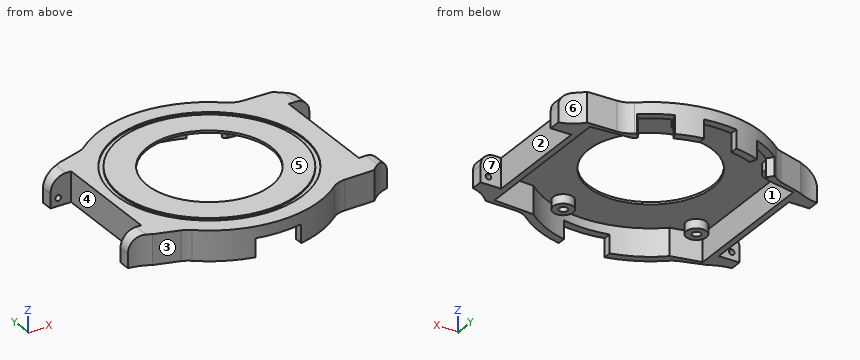
```python
from build123d import *

# Parameters (mm, degrees)
PAD_DEPTH       = 6.5
POCKET_DEPTH    = 6
SKETCH002_R     = 13.5
POCKET001_DEPTH = 1
SKETCH003_W     = 5.4
SKETCH003_H     = 6.5
PAD001_DEPTH    = 4.5
POCKET002_DEPTH = 10
SKETCH008_R     = 0.6
POCKET003_DEPTH = 2
SKETCH009_R     = 0.6
POCKET004_DEPTH = 2
FILLET_R        = 2.9
FILLET001_R     = 2.9
FILLET002_R     = 5
FILLET003_R     = 5
FILLET004_R     = 5
FILLET005_R     = 5
SKETCH010_W     = 3.95
SKETCH010_H     = 6.5
PAD002_DEPTH    = 4.5
POCKET005_DEPTH = 10
SKETCH012_R     = 0.6
POCKET006_DEPTH = 2
SKETCH013_R     = 0.6
POCKET007_DEPTH = 2
FILLET006_R     = 3.4
FILLET007_R     = 3.4
SKETCH014_R     = 20.45
SKETCH014_R_2   = 19.5
POCKET008_DEPTH = 0.3
SKETCH015_R     = 2.2
SKETCH015_R_2   = 0.925
PAD003_DEPTH    = 2
POCKET009_DEPTH = 4
POCKET010_DEPTH = 4


with BuildPart() as part:
    # Sketch → Pad (new body)
    with BuildSketch(Plane.XY):
        with BuildLine():
            Line((-22.5019915649, 16), (-22.5019915649, -16))
            Line((-22.5019915649, -16), (-16.2858834578, -17.9000000001))
            ThreePointArc((-16.2858834577, -17.9000000001), (0.2206895737, -24.1989937004), (16.6096357576, -17.5999999999))
            Line((16.6096357576, -17.5999999999), (24.9082802252, -17.45))
            Line((24.9082802252, 17.45), (24.9082802252, -17.45))
            Line((16.6096357576, 17.6), (24.9082802252, 17.45))
            ThreePointArc((16.6096357576, 17.6), (0.2206895736, 24.1989937004), (-16.2858834578, 17.9))
            Line((-22.5019915649, 16), (-16.2858834578, 17.9))
        make_face()
    extrude(amount=PAD_DEPTH)

    # Sketch001 → Pocket (cut)
    with BuildSketch(Plane.XY):
        with BuildLine():
            Line((-14.8539557021, 16.9), (-21.2122180433, 15.55))
            Line((-21.2122180433, 15.55), (-21.2122180433, -15.55))
            Line((-21.2122180433, -15.55), (-14.8539557021, -16.9))
            ThreePointArc((-14.8539557021, -16.9), (-0.0760301383, -22.4998715423), (14.739402973, -17))
            Line((14.739402973, -17), (23.6191552218, -16.4))
            Line((23.6191552218, 16.4), (23.6191552218, -16.4))
            Line((14.739402973, 17), (23.6191552218, 16.4))
            ThreePointArc((14.739402973, 17), (-0.0760301383, 22.4998715423), (-14.8539557021, 16.9))
        make_face()
    extrude(amount=POCKET_DEPTH, mode=Mode.SUBTRACT)

    # Sketch002 (on Face19 of Pocket) → Pocket001 (cut)
    with BuildSketch(Plane(origin=(0, 0, 6), x_dir=(1, 0, 0), z_dir=(0, 0, -1))):
        Circle(SKETCH002_R)
    extrude(amount=-POCKET001_DEPTH, mode=Mode.SUBTRACT)

    # Sketch003 (on Face6 of Pocket001) → Pad001 (join)
    with BuildSketch(Plane.YZ.offset(24.9082802252)):
        with Locations((-14.75, 3.25)):
            Rectangle(SKETCH003_W, SKETCH003_H)
        with Locations((14.75, 3.25)):
            Rectangle(SKETCH003_W, SKETCH003_H)
    extrude(amount=PAD001_DEPTH)

    # Sketch006 → Pocket002 (cut)
    with BuildSketch(Plane.XY.offset(6.5)):
        with BuildLine():
            ThreePointArc((24.9082802253, 17.45), (26.9423471239, 15.7065020586), (29.4082802252, 14.6594169812))
            Line((29.4082802252, 17.45), (29.4082802252, 14.6594169812))
            Line((29.4082802252, 17.45), (24.9082802252, 17.45))
        make_face()
        with BuildLine():
            ThreePointArc((29.4082802253, -14.6594169812), (26.9423471239, -15.7065020586), (24.9082802253, -17.45))
            Line((29.4082802252, -17.45), (24.9082802252, -17.45))
            Line((29.4082802253, -14.6594169811), (29.4082802252, -17.45))
        make_face()
    extrude(amount=-POCKET002_DEPTH, mode=Mode.SUBTRACT)

    # Sketch008 (on Face27 of Pocket002) → Pocket003 (cut)
    with BuildSketch(Plane(origin=(0, -12.05, 0), x_dir=(-1, 0, 0), z_dir=(0, 1, 0))):
        with Locations((-27.7082802252, 1.7)):
            Circle(SKETCH008_R)
    extrude(amount=-POCKET003_DEPTH, mode=Mode.SUBTRACT)

    # Sketch009 (on Face26 of Pocket003) → Pocket004 (cut)
    with BuildSketch(Plane.XZ.offset(-12.05)):
        with Locations((27.7082802252, 1.7)):
            Circle(SKETCH009_R)
    extrude(amount=-POCKET004_DEPTH, mode=Mode.SUBTRACT)

    # Fillet
    fillet_edges = [part.edges().sort_by_distance(p)[0] for p in [
        (29.40828, -13.354708, 6.5),
    ]]
    fillet(fillet_edges, radius=FILLET_R)

    # Fillet001
    fillet001_edges = [part.edges().sort_by_distance(p)[0] for p in [
        (29.40828, 13.354708, 6.5),
    ]]
    fillet(fillet001_edges, radius=FILLET001_R)

    # Fillet002
    fillet002_edges = [part.edges().sort_by_distance(p)[0] for p in [
        (16.609636, -17.6, 3.25),
    ]]
    fillet(fillet002_edges, radius=FILLET002_R)

    # Fillet003
    fillet003_edges = [part.edges().sort_by_distance(p)[0] for p in [
        (16.609636, 17.6, 3.25),
    ]]
    fillet(fillet003_edges, radius=FILLET003_R)

    # Fillet004
    fillet004_edges = [part.edges().sort_by_distance(p)[0] for p in [
        (-16.285883, -17.9, 3.25),
    ]]
    fillet(fillet004_edges, radius=FILLET004_R)

    # Fillet005
    fillet005_edges = [part.edges().sort_by_distance(p)[0] for p in [
        (-16.285883, 17.9, 3.25),
    ]]
    fillet(fillet005_edges, radius=FILLET005_R)

    # Sketch010 (on Face4 of Fillet005) → Pad002 (join)
    with BuildSketch(Plane(origin=(-22.5019915649, 0, 0), x_dir=(0, -1, 0), z_dir=(-1, 0, 0))):
        with Locations((-14.025, 3.25)):
            Rectangle(SKETCH010_W, SKETCH010_H)
        with Locations((14.025, 3.25)):
            Rectangle(SKETCH010_W, SKETCH010_H)
    extrude(amount=PAD002_DEPTH)

    # Sketch011 (on Face6 of Pad002) → Pocket005 (cut)
    with BuildSketch(Plane.XY.offset(6.5)):
        with BuildLine():
            ThreePointArc((-27.0019915649, 14.6), (-24.6759937451, 15.0557212933), (-22.5019915649, 16))
            Line((-22.5019915649, 16), (-27.0019915649, 16))
            Line((-27.0019915649, 16), (-27.0019915649, 14.6))
        make_face()
        with BuildLine():
            ThreePointArc((-22.5019915649, -16), (-24.6759937451, -15.0557212933), (-27.0019915649, -14.6))
            Line((-27.0019915649, -14.6), (-27.0019915649, -16))
            Line((-27.0019915649, -16), (-22.5019915649, -16))
        make_face()
    extrude(amount=-POCKET005_DEPTH, mode=Mode.SUBTRACT)

    # Sketch012 (on Face23 of Pocket005) → Pocket006 (cut)
    with BuildSketch(Plane(origin=(0, -12.05, 0), x_dir=(-1, 0, 0), z_dir=(0, 1, 0))):
        with Locations((25.3019915649, 1.7)):
            Circle(SKETCH012_R)
    extrude(amount=-POCKET006_DEPTH, mode=Mode.SUBTRACT)

    # Sketch013 (on Face21 of Pocket006) → Pocket007 (cut)
    with BuildSketch(Plane.XZ.offset(-12.05)):
        with Locations((-25.3019915649, 1.7)):
            Circle(SKETCH013_R)
    extrude(amount=-POCKET007_DEPTH, mode=Mode.SUBTRACT)

    # Fillet006
    fillet006_edges = [part.edges().sort_by_distance(p)[0] for p in [
        (-27.001992, 13.325, 6.5),
    ]]
    fillet(fillet006_edges, radius=FILLET006_R)

    # Fillet007
    fillet007_edges = [part.edges().sort_by_distance(p)[0] for p in [
        (-27.001992, -13.325, 6.5),
    ]]
    fillet(fillet007_edges, radius=FILLET007_R)

    # Sketch014 (on Face4 of Fillet007) → Pocket008 (cut)
    with BuildSketch(Plane.XY.offset(6.5)):
        Circle(SKETCH014_R)
        Circle(SKETCH014_R_2, mode=Mode.SUBTRACT)
    extrude(amount=-POCKET008_DEPTH, mode=Mode.SUBTRACT)

    # Sketch015 (on Face55 of Pocket008) → Pad003 (join)
    with BuildSketch(Plane(origin=(0, 0, 6), x_dir=(1, 0, 0), z_dir=(0, 0, -1))):
        with Locations((-18.42, 13.32)):
            Circle(SKETCH015_R)
        with Locations((-18.42, 13.32)):
            Circle(SKETCH015_R_2, mode=Mode.SUBTRACT)
        with Locations((7.27, 18.56)):
            Circle(SKETCH015_R)
        with Locations((7.27, 18.56)):
            Circle(SKETCH015_R_2, mode=Mode.SUBTRACT)
        with Locations((5.37, -19.79)):
            Circle(SKETCH015_R)
        with Locations((5.37, -19.79)):
            Circle(SKETCH015_R_2, mode=Mode.SUBTRACT)
        with Locations((-18.42, -13.32)):
            Circle(SKETCH015_R)
        with Locations((-18.42, -13.32)):
            Circle(SKETCH015_R_2, mode=Mode.SUBTRACT)
    extrude(amount=PAD003_DEPTH)

    # Sketch016 → Pocket009 (cut)
    with BuildSketch(Plane(origin=(0, 0, 0), x_dir=(-1, 0, 0), z_dir=(0, 0, 1))):
        with BuildLine():
            Line((-5, 23.6778377391), (-5, 21.9374109685))
            ThreePointArc((5, 21.9374109685), (0, 22.5), (-5, 21.9374109685))
            Line((5, 23.6778377391), (5, 21.9374109685))
            ThreePointArc((5, 23.6778377391), (0, 24.2), (-5, 23.6778377391))
        make_face()
    extrude(amount=POCKET009_DEPTH, mode=Mode.SUBTRACT)

    # Sketch017 → Pocket010 (cut)
    with BuildSketch(Plane(origin=(0, 0, 0), x_dir=(-1, 0, 0), z_dir=(0, 0, 1))):
        with BuildLine():
            Line((-3.499984119, -22.2261132717), (-3.5, -23.9455632634))
            ThreePointArc((-3.5, -23.9455632634), (0, -24.2000019575), (3.5, -23.9455632634))
            Line((3.5000158811, -22.2261082701), (3.5, -23.9455632634))
            ThreePointArc((-3.499984119, -22.2261132717), (1.60767e-05, -22.5), (3.5000158811, -22.2261082701))
        make_face()
        with BuildLine():
            ThreePointArc((-13.9498796389, -17.6536358312), (-11.25, -19.4855715851), (-8.3135572795, -20.9077680626))
            Line((-8.3135572795, -20.9077680626), (-8.9416927184, -22.487466094))
            ThreePointArc((-15.0038705449, -18.987466094), (-12.1, -20.9578147716), (-8.9416927184, -22.487466094))
            Line((-13.9498796389, -17.6536358312), (-15.0038705449, -18.987466094))
        make_face()
        with BuildLine():
            ThreePointArc((8.3135572795, -20.9077680626), (11.25, -19.4855715851), (13.9498796389, -17.6536358312))
            Line((13.9498796389, -17.6536358312), (15.0038705449, -18.987466094))
            ThreePointArc((8.9416927184, -22.487466094), (12.1, -20.9578147716), (15.0038705449, -18.987466094))
            Line((8.3135572795, -20.9077680626), (8.9416927184, -22.487466094))
        make_face()
    extrude(amount=POCKET010_DEPTH, mode=Mode.SUBTRACT)


solid = part.part
```
CAD build for the part. Positions are in the model's coordinates, mm. Face numbers are marked on the shaded views. A direction names the side the tool comes from. Give positions to 0.01 mm unless a question says otherwise; leave off trailing zeros. Loops run counter-clockwise (first coordinate to the right, second up) from the corner with the lowest first, then second, coordinate; pieces in that order, holes last. Notation, with made-up numbers: (36, 88.25) - (48, 88.25) arc R11 cw to (48, 93.25) - close; hole circle Ø1 at (81, 55). An arc over 180 degrees is marked (long way). Put each result on its own line as item: value.
Q1. Slice it at B-B (y = 0). Give the cut face in (x, z).
Filled in:
outline: (-22.5, 0) - (-21.21, 0) - (-21.21, 6) - (-13.5, 6) - (-13.5, 6.5) - (-19.5, 6.5) - (-19.5, 6.2) - (-20.45, 6.2) - (-20.45, 6.5) - (-22.5, 6.5) - close; (13.5, 6) - (23.62, 6) - (23.62, 0) - (24.91, 0) - (24.91, 6.5) - (20.45, 6.5) - (20.45, 6.2) - (19.5, 6.2) - (19.5, 6.5) - (13.5, 6.5) - close
Q2. Probe line 1 along X through (y, z) = (7, 1.25); line 2 along Y through (x, z) = (-18.42, 5.65) (3 decimals); line 3 along Y through (x, z) = (-23, 4.25). List the from-to ranges inside material, lowest first.
Filled in:
line 1: x = -22.5 to -21.21, 23.62 to 24.91
line 2: y = -17.248 to -16.143, -15.52 to -14.245, -12.395 to -11.12, 11.12 to 12.395, 14.245 to 15.52, 16.143 to 17.248
line 3: y = -15.73 to -12.05, 12.05 to 15.73
Q3. Flat gauge pins, fed straight in: pin 1 (1.5 mm diameter, centred on x = 22.5, y = -6.5, fed in from -Z); pin 2 (2 mm diameter, centred on x = -18.5, y = 13.5, fed in from -Z); pin 3 (3.5 mm diameter, centred on x = -24, z = 2.5, fed in from +Y). Where does each tip first touch, or does it go through?
Filled in:
pin 1: stops at z = 6
pin 2: stops at z = 4
pin 3: stops at y = 16.08
Q4. Slice it at C-C (z = 5.25). Give the number of separate pieces and of enclosed holes in the cut face, plus the area to 3 significant figures.
Filled in:
separate pieces: 4
enclosed holes: 5
area: 334 mm²
Q5. Slice it at A-A (x = 0). Give the cut face in (y, z).
Filled in:
outline: (-24.2, 4) - (-22.5, 4) - (-22.5, 6) - (-13.5, 6) - (-13.5, 6.5) - (-19.5, 6.5) - (-19.5, 6.2) - (-20.45, 6.2) - (-20.45, 6.5) - (-24.2, 6.5) - close; (13.5, 6) - (22.5, 6) - (22.5, 4) - (24.2, 4) - (24.2, 6.5) - (20.45, 6.5) - (20.45, 6.2) - (19.5, 6.2) - (19.5, 6.5) - (13.5, 6.5) - close
Q6. Tool access for the marked faces 1, 2, 3 and 4: list every direction of +Z, -Z, +X, -X, +Y, -Y with a clear straight run to the whole face (end or side of a thin tool).
Filled in:
face 1: -Z
face 2: +Z, -Z, +X
face 3: +Z, -Z, -X, -Y
face 4: +Z, -Z, -X
Q7. Mould opens along Y. For the marked faces 5, 6 and 7 say: pulls with the +Y half, pulls with the -Y half, needs draft (parallel to the pull), parting line crosses it, or undercut.
Filled in:
face 5: needs draft
face 6: pulls with the +Y half
face 7: undercut
